```python
from build123d import *

# Parameters (mm, degrees)
SKETCH1_R           = 18
BOSS_EXTRUDE1_DEPTH = 60
SKETCH2_R           = 8
BOSS_EXTRUDE2_DEPTH = 3
SKETCH3_R           = 16
BOSS_EXTRUDE3_DEPTH = 39
BOSS_EXTRUDE4_DEPTH = 3
BOSS_EXTRUDE5_DEPTH = 16


with BuildPart() as part:
    # Sketch1 → Boss-Extrude1 (new body)
    with BuildSketch(Plane(origin=(0, 0, 0), x_dir=(0, 0, -1), z_dir=(1, 0, 0))):
        Circle(SKETCH1_R)
    extrude(amount=BOSS_EXTRUDE1_DEPTH)

    # Sketch2 → Boss-Extrude2 (add)
    with BuildSketch(Plane.ZY):
        Circle(SKETCH2_R)
    extrude(amount=BOSS_EXTRUDE2_DEPTH)

    # Sketch3 → Boss-Extrude3 (add)
    with BuildSketch(Plane(origin=(60, 0, 0), x_dir=(0, 0, -1), z_dir=(1, 0, 0))):
        Circle(SKETCH3_R)
    extrude(amount=BOSS_EXTRUDE3_DEPTH)

    # Sketch4 → Boss-Extrude4 (add)
    with BuildSketch(Plane(origin=(99, 0, 0), x_dir=(0, 0, -1), z_dir=(1, 0, 0))):
        with BuildLine():
            Line((9, 4.358898944), (9, -4.358898944))
            ThreePointArc((9, -4.358898944), (0, -10), (-9, -4.358898944))
            Line((-9, -4.358898944), (-9, 4.358898944))
            ThreePointArc((-9, 4.358898944), (0, 10), (9, 4.358898944))
        make_face()
    extrude(amount=BOSS_EXTRUDE4_DEPTH)

    # Sketch5 → Boss-Extrude5 (add)
    with BuildSketch(Plane(origin=(102, 0, 0), x_dir=(0, 0, -1), z_dir=(1, 0, 0))):
        with BuildLine():
            Line((-1.658312395, 2.5), (1.658312395, 2.5))
            ThreePointArc((1.658312395, 2.5), (0, -3), (-1.658312395, 2.5))
        make_face()
    extrude(amount=BOSS_EXTRUDE5_DEPTH)


solid = part.part
```
Could you check a few things on this model? Use its own coordinates, in mm. A direction names the side the tool comes from. Round coordinates to 2 decimals unless told otherwise and drop trailing zeros. Write each loop counter-clockwise with the first axis right and the second up, starting at its lowest first coordinate (ties: lowest second). Pieces come first, ordered by that corner, then holes. Notation, with made-up numbers: M 81.5,-23.5 L 109.5,-23.5 A11 cw 109.5,-5.5 Z; hole C -26,-36 d8. An arc over 180 degrees is marked long. Answer in a Markdown table with one row per item. Add a question column.
Q1. Imagine slicing it at D-D (y = 11.5). Please give me the cut outline in (x, z).
Q2. Imagine slicing it at A-A (z = 0). Please give me the cut outline in (x, y), then the cut area to 3 significant figures.
Q3. If I drill on line 1 (X direction, y = 10.5, z = -3); line 2 (X direction, y = -6, z = 1); line 3 (Y direction, x = 37.5, z = 0), over which ranges is the centre line in solid material (lowest first)? Write a range as from..to.
Q4. Imagine slicing it at B-B (y = 0). Please give me the cut outline in (x, z), then the cut area to 3 significant figures.
Q5. Imagine slicing it at C-C (x = 23.5). Please give me the cut outline in (y, z), then the cut area to 3 significant figures.
Q6. Will these pins go through, and if not, where does the flat tip stop? pin 1 Ø3 at (x, y) = (78, -1) entering from -Z; pin 2 Ø2 at (x, z) = (31.5, -6.5) entering from -Y; pin 3 Ø1.5 at (y, z) = (-11.5, 3) entering from -X.
Q7. On a 3-axis mill with a long thin cutter (end or side, diameter ignored), from which of +Z, -Z, +X, -X, +Y, -Y can I reach the whole of each face in a straight line? I mean faces 1 (the flat face through (0, -4, -8)), 2 (the flat face through (100, 0, 9)), 3 (the flat face through (99, 0, -10)), 4 (the cylindrical face through (100, 10, 0)). Say none if no direction works.
Values:
| question | item | result |
|---|---|---|
| 1 | outline | M 0,-13.85 L 60,-13.85 L 60,-11.12 L 99,-11.12 L 99,11.12 L 60,11.12 L 60,13.85 L 0,13.85 Z |
| 2 | outline | M -3,-8 L 0,-8 L 0,-18 L 60,-18 L 60,-16 L 99,-16 L 99,-10 L 102,-10 L 102,-3 L 118,-3 L 118,2.5 L 102,2.5 L 102,10 L 99,10 L 99,16 L 60,16 L 60,18 L 0,18 L 0,8 L -3,8 Z |
| 2 | area | 3,600 mm^2 |
| 3 | line 1 | 0..99 |
| 3 | line 2 | -3..102 |
| 3 | line 3 | -18..18 |
| 4 | outline | M -3,-8 L 0,-8 L 0,-18 L 60,-18 L 60,-16 L 99,-16 L 99,-9 L 102,-9 L 102,-3 L 118,-3 L 118,3 L 102,3 L 102,9 L 99,9 L 99,16 L 60,16 L 60,18 L 0,18 L 0,8 L -3,8 Z |
| 4 | area | 3,610 mm^2 |
| 5 | outline | C 0,0 d36 |
| 5 | area | 1,020 mm^2 |
| 6 | pin 1 | z = -16 |
| 6 | pin 2 | y = -17.14 |
| 6 | pin 3 | x = 0 |
| 7 | face 1 | -X |
| 7 | face 2 | +Z, +X, +Y, -Y |
| 7 | face 3 | +X |
| 7 | face 4 | +X, +Y |
